Source: CAD feature listing. Evaluate the final solid. Frame: model axes, mm. Face numbers are marked on the shaded views. A direction names the side the tool comes from. Coordinates: 2 decimals unless noted, no trailing zeros. Order: outer loops, then holes, each group sorted by start corner. A loop starts at its lowest first (then second) coordinate and runs counter-clockwise, first axis right, second up.
```python
from build123d import *

# Parameters (mm, degrees)
BOSS_EXTRU_1_DEPTH      = 30
ESQUISSE3_W             = 6.5
ESQUISSE3_H             = 96
ENL_V_MAT_EXTRU_1_DEPTH = 11.5
ENL_V_START             = -5.5
ENL_V_MAT_EXTRU_2_DEPTH = 5.5
ENL_V_MAT_EXTRU_3_DEPTH = 5.5
ENL_V_MAT_EXTRU_4_DEPTH = 2
ENL_V_MAT_EXTRU_5_DEPTH = 2
CONG_2_R                = 2.5
CONG_3_R                = 2.5
CONG_4_R                = 2.5
CONG_5_R                = 2.5


with BuildPart() as part:
    # Esquisse1 → Boss.-Extru.1 (new body)
    with BuildSketch(Plane.XY):
        Polygon((-35.56359131, -94.611176471), (-35.56359131, 1.388823529), (108.43640869, 1.388823529), (108.43640869, -8.611176471), (90.581116466, -34.111176471), (77.93640869, -34.111176471), (77.93640869, -59.111176471), (87.721135464, -59.111176471), (105.576427689, -84.611176471), (105.576427689, -94.611176471), align=None)
        with BuildLine():
            Line((-5.06359131, -21.611176471), (46.93640869, -21.611176471))
            ThreePointArc((46.93640869, -21.611176471), (52.43640869, -16.111176471), (46.93640869, -10.611176471))
            Line((46.93640869, -10.611176471), (-5.06359131, -10.611176471))
            ThreePointArc((-5.06359131, -10.611176471), (-10.56359131, -16.111176471), (-5.06359131, -21.611176471))
        make_face(mode=Mode.SUBTRACT)
        with BuildLine():
            Line((-5.06359131, -82.611176471), (46.93640869, -82.611176471))
            ThreePointArc((46.93640869, -82.611176471), (52.43640869, -77.111176471), (46.93640869, -71.611176471))
            Line((46.93640869, -71.611176471), (-5.06359131, -71.611176471))
            ThreePointArc((-5.06359131, -71.611176471), (-10.56359131, -77.111176471), (-5.06359131, -82.611176471))
        make_face(mode=Mode.SUBTRACT)
    extrude(amount=BOSS_EXTRU_1_DEPTH)

    # Esquisse3 → Enlèv. mat.-Extru.1 (cut)
    with BuildSketch(Plane.XY.offset(30)):
        with Locations((-32.31359131, -46.611176471)):
            Rectangle(ESQUISSE3_W, ESQUISSE3_H)
    extrude(amount=-ENL_V_MAT_EXTRU_1_DEPTH, mode=Mode.SUBTRACT)

    # Esquisse4 → Enlèv. mat.-Extru.2 (cut)
    # profile 1 of 2: a face of its own
    with BuildSketch(Plane.XY.offset(30).offset(ENL_V_START)):
        Polygon((-29.06359131, 1.388823529), (-29.06359131, -34.111176471), (77.93640869, -34.111176471), (90.581116466, -34.111176471), (103.534955923, -15.611176471), (73.43640869, -15.611176471), (73.43640869, 1.388823529), align=None)
        with BuildLine():
            ThreePointArc((46.93640869, -10.611176471), (52.43640869, -16.111176471), (46.93640869, -21.611176471))
            Line((46.93640869, -21.611176471), (-5.06359131, -21.611176471))
            ThreePointArc((-5.06359131, -21.611176471), (-10.56359131, -16.111176471), (-5.06359131, -10.611176471))
            Line((-5.06359131, -10.611176471), (46.93640869, -10.611176471))
        make_face(mode=Mode.SUBTRACT)
    # profile 2 of 2: a face of its own
    with BuildSketch(Plane.XY.offset(30).offset(ENL_V_START)):
        Polygon((-29.06359131, -94.611176471), (70.576427689, -94.611176471), (70.576427689, -77.611176471), (100.674974921, -77.611176471), (87.721135464, -59.111176471), (77.93640869, -59.111176471), (-29.06359131, -59.111176471), align=None)
        with BuildLine():
            ThreePointArc((46.93640869, -71.611176471), (52.43640869, -77.111176471), (46.93640869, -82.611176471))
            Line((46.93640869, -82.611176471), (-5.06359131, -82.611176471))
            ThreePointArc((-5.06359131, -82.611176471), (-10.56359131, -77.111176471), (-5.06359131, -71.611176471))
            Line((-5.06359131, -71.611176471), (46.93640869, -71.611176471))
        make_face(mode=Mode.SUBTRACT)
    extrude(amount=ENL_V_MAT_EXTRU_2_DEPTH, mode=Mode.SUBTRACT)

    # Esquisse5 → Enlèv. mat.-Extru.3 (cut)
    # profile 1 of 2: a face of its own
    with BuildSketch(Plane(origin=(0, 0, 0), x_dir=(-1, 0, 0), z_dir=(0, 0, -1))):
        Polygon((-73.43640869, -15.611176471), (-103.534955923, -15.611176471), (-90.581116466, -34.111176471), (-77.93640869, -34.111176471), (29.06359131, -34.111176471), (29.06359131, 1.388823529), (-73.43640869, 1.388823529), align=None)
        with BuildLine():
            ThreePointArc((5.06359131, -10.611176471), (10.56359131, -16.111176471), (5.06359131, -21.611176471))
            Line((5.06359131, -21.611176471), (-46.93640869, -21.611176471))
            ThreePointArc((-46.93640869, -21.611176471), (-52.43640869, -16.111176471), (-46.93640869, -10.611176471))
            Line((-46.93640869, -10.611176471), (5.06359131, -10.611176471))
        make_face(mode=Mode.SUBTRACT)
    # profile 2 of 2: a face of its own
    with BuildSketch(Plane(origin=(0, 0, 0), x_dir=(-1, 0, 0), z_dir=(0, 0, -1))):
        Polygon((-77.93640869, -59.111176471), (-87.721135464, -59.111176471), (-100.674974921, -77.611176471), (-70.576427689, -77.611176471), (-70.576427689, -94.611176471), (29.06359131, -94.611176471), (29.06359131, -59.111176471), align=None)
        with BuildLine():
            ThreePointArc((5.06359131, -71.611176471), (10.56359131, -77.111176471), (5.06359131, -82.611176471))
            Line((5.06359131, -82.611176471), (-46.93640869, -82.611176471))
            ThreePointArc((-46.93640869, -82.611176471), (-52.43640869, -77.111176471), (-46.93640869, -71.611176471))
            Line((-46.93640869, -71.611176471), (5.06359131, -71.611176471))
        make_face(mode=Mode.SUBTRACT)
    extrude(amount=-ENL_V_MAT_EXTRU_3_DEPTH, mode=Mode.SUBTRACT)

    # Esquisse6 → Enlèv. mat.-Extru.4 (cut)
    with BuildSketch(Plane(origin=(0, 0, 0), x_dir=(-1, 0, 0), z_dir=(0, 0, -1))):
        Polygon((-103.534955923, -15.611176471), (-73.43640869, -15.611176471), (-73.43640869, 1.388823529), (-108.43640869, 1.388823529), (-108.43640869, -8.611176471), align=None)
        Polygon((-70.576427689, -77.611176471), (-100.674974921, -77.611176471), (-105.576427689, -84.611176471), (-105.576427689, -94.611176471), (-70.576427689, -94.611176471), align=None)
    extrude(amount=-ENL_V_MAT_EXTRU_4_DEPTH, mode=Mode.SUBTRACT)

    # Esquisse7 → Enlèv. mat.-Extru.5 (cut)
    with BuildSketch(Plane.XY.offset(30)):
        Polygon((73.43640869, -15.611176471), (103.534955923, -15.611176471), (108.43640869, -8.611176471), (108.43640869, 1.388823529), (73.43640869, 1.388823529), align=None)
        Polygon((100.674974921, -77.611176471), (70.576427689, -77.611176471), (70.576427689, -94.611176471), (105.576427689, -94.611176471), (105.576427689, -84.611176471), align=None)
    extrude(amount=-ENL_V_MAT_EXTRU_5_DEPTH, mode=Mode.SUBTRACT)

    # Congé2
    cong_2_edges = [part.edges().sort_by_distance(p)[0] for p in [
        (20.93640869, -10.611176471, 24.5),
        (-10.56359131, -16.111176471, 24.5),
        (20.93640869, -21.611176471, 24.5),
        (52.43640869, -16.111176471, 24.5),
    ]]
    fillet(cong_2_edges, radius=CONG_2_R)

    # Congé3
    cong_3_edges = [part.edges().sort_by_distance(p)[0] for p in [
        (52.43640869, -77.111176471, 24.5),
        (20.93640869, -71.611176471, 24.5),
        (-10.56359131, -77.111176471, 24.5),
        (20.93640869, -82.611176471, 24.5),
    ]]
    fillet(cong_3_edges, radius=CONG_3_R)

    # Congé4
    cong_4_edges = [part.edges().sort_by_distance(p)[0] for p in [
        (-10.56359131, -16.111176471, 5.5),
        (20.93640869, -10.611176471, 5.5),
        (52.43640869, -16.111176471, 5.5),
        (20.93640869, -21.611176471, 5.5),
    ]]
    fillet(cong_4_edges, radius=CONG_4_R)

    # Congé5
    cong_5_edges = [part.edges().sort_by_distance(p)[0] for p in [
        (-10.56359131, -77.111176471, 5.5),
        (20.93640869, -71.611176471, 5.5),
        (52.43640869, -77.111176471, 5.5),
        (20.93640869, -82.611176471, 5.5),
    ]]
    fillet(cong_5_edges, radius=CONG_5_R)


solid = part.part
```
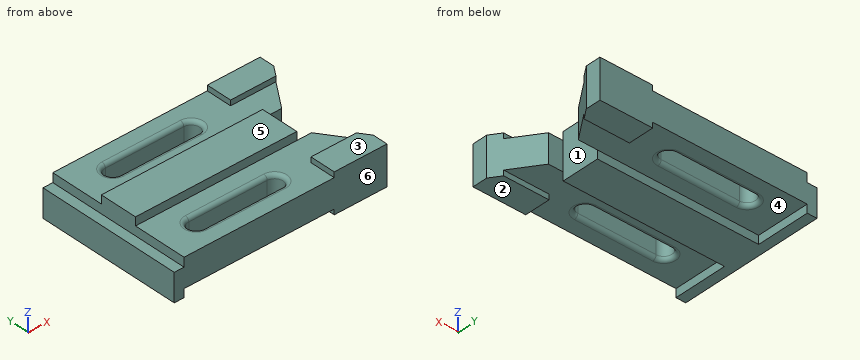
1. Section query A-A, the plane z = 3.5. Output: boundary loops of the cut face in (x, y), plus the area to 3 significant figures.
2. Access query for the marked faces 1, 2 and 3. Directions: +Z, -Z, +X, -X, +Y, -Y. A direction counts if a zero-diameter tool reaches every point of the face in a straight line with its end or side. Return the directions, or none.
3. Section query B-B, the plane x = 27. Output: boundary loops of the cut face in (y, z), plus the area to 3 significant figures.
4. Section query D-D, the plane y = -37. Output: boundary loops of the cut face in (x, z).
5. Material intervals for line 1 along X through (y, z) = (-85, 3.75); line 2 along Y through (x, z) = (29, 12.25); line 3 along Y through (x, z) = (-5, 23.5), sorted ascending.
6. Contact query for flat-ended pins moving along their axis: P1, Ø10, axis at x = 3, y = -69.5, coming from the +Z side; P2, Ø12, axis at y = -31, z = 15.5, coming from the +X side; P3, Ø1, axis at x = -14, y = -36.5, coming from the -Z side; P4, Ø2, axis at x = -32, y = -34, coming from the +Z side. Output: stop coordinate, or through.
7. Draft query along Y for the marked faces 4, 5 and 6. Return one class per face: +Y half, -Y half, draft (parallel to the pull), parting line (faces both ways), or undercut.
8. Section query C-C, the plane z = 10.25. Output: boundary loops of the cut face in (x, y).
Answer key:
1. outline: (-35.56, -94.61) - (-29.06, -94.61) - (-29.06, -59.11) - (77.94, -59.11) - (77.94, -34.11) - (-29.06, -34.11) - (-29.06, 1.39) - (-35.56, 1.39) - close; (70.58, -94.61) - (105.58, -94.61) - (105.58, -84.61) - (100.67, -77.61) - (70.58, -77.61) - close; (73.44, -15.61) - (103.53, -15.61) - (108.44, -8.61) - (108.44, 1.39) - (73.44, 1.39) - close
1. area: 4,450 mm2
2. face 1: +Z, -Z, +X
2. face 2: -Z, +X, -Y
2. face 3: +Z, +X, -X, -Y
3. outline: (-94.61, 5.5) - (-85.11, 5.5) arc R2.5 ccw to (-82.61, 8) - (-82.61, 22) arc R2.5 ccw to (-85.11, 24.5) - (-94.61, 24.5) - close; (-71.61, 8) arc R2.5 ccw to (-69.11, 5.5) - (-59.11, 5.5) - (-59.11, 0) - (-34.11, 0) - (-34.11, 5.5) - (-24.11, 5.5) arc R2.5 ccw to (-21.61, 8) - (-21.61, 22) arc R2.5 ccw to (-24.11, 24.5) - (-34.11, 24.5) - (-34.11, 30) - (-59.11, 30) - (-59.11, 24.5) - (-69.11, 24.5) arc R2.5 ccw to (-71.61, 22) - close; (-10.61, 8) arc R2.5 ccw to (-8.11, 5.5) - (1.39, 5.5) - (1.39, 24.5) - (-8.11, 24.5) arc R2.5 ccw to (-10.61, 22) - close
3. area: 1,670 mm2
4. outline: (-35.56, 0) - (77.94, 0) - (77.94, 30) - (-29.06, 30) - (-29.06, 18.5) - (-35.56, 18.5) - close
5. line 1: x = -35.56 to -29.06, 70.58 to 105.58
5. line 2: y = -94.61 to -82.61, -71.61 to -21.61, -10.61 to 1.39
5. line 3: y = -94.61 to -83.11, -71.11 to -22.11, -10.11 to 1.39
6. P1: stops at z = 24.5
6. P2: stops at x = 96.96
6. P3: stops at z = 0
6. P4: stops at z = 18.5
7. face 4: undercut
7. face 5: draft
7. face 6: -Y half
8. outline: (-35.56, -94.61) - (105.58, -94.61) - (105.58, -84.61) - (87.72, -59.11) - (77.94, -59.11) - (77.94, -34.11) - (90.58, -34.11) - (108.44, -8.61) - (108.44, 1.39) - (-35.56, 1.39) - close; hole (-5.06, -82.61) - (46.94, -82.61) arc R5.5 ccw to (46.94, -71.61) - (-5.06, -71.61) arc R5.5 ccw to start; hole (-5.06, -21.61) - (46.94, -21.61) arc R5.5 ccw to (46.94, -10.61) - (-5.06, -10.61) arc R5.5 ccw to start
